from build123d import *

# Parameters (mm, degrees)
F0_W     = 110.9530478716
F0_H     = 111.6942763329
F1_DEPTH = 55.1221389323
F1_TAPER = 3
F2_R     = 10.16
F3_T     = -2.54
F4_R     = 11.5246315094
F4_R_2   = 8.0655463765
F5_DEPTH = 25.4
F6_DEPTH = 25.4


with BuildPart() as f1:
    # F0 (on Top) → F1 (new body)
    with BuildSketch(Plane.XY):
        Rectangle(F0_W, F0_H)
    extrude(amount=F1_DEPTH, taper=F1_TAPER)

    # F2
    f2_edges = [f1.edges().sort_by_distance(p)[0] for p in [
        (54.032109, -54.402724, 27.561069),
        (52.587695, 0, 55.122139),
        (0, -52.958309, 55.122139),
        (54.032109, 54.402724, 27.561069),
        (0, 52.958309, 55.122139),
        (-54.032109, 54.402724, 27.561069),
        (-52.587695, 0, 55.122139),
        (-54.032109, -54.402724, 27.561069),
    ]]
    fillet(f2_edges, radius=F2_R)

    # F3
    f3_openings = [f1.faces().sort_by_distance(p)[0] for p in [
        (0, 0, 0),
    ]]
    offset(amount=F3_T, openings=f3_openings)

    # F4 (on face) → F5 (join)
    with BuildSketch(Plane(origin=(0, 0, 52.5821389323), x_dir=(1, 0, 0), z_dir=(0, 0, -1))):
        with Locations((24.3312865496, -14.7694125772)):
            Circle(F4_R)
        with Locations((24.3312865496, -14.7694125772)):
            Circle(F4_R_2, mode=Mode.SUBTRACT)
    extrude(amount=F5_DEPTH)

    # F6 (cut): a face of the model
    f6_faces = [f1.faces().sort_by_distance(p)[0] for p in [
        (24.3312865496, 14.7694125772, 52.5821389323),
    ]]
    extrude(f6_faces, amount=-F6_DEPTH, mode=Mode.SUBTRACT)


solid = f1.part
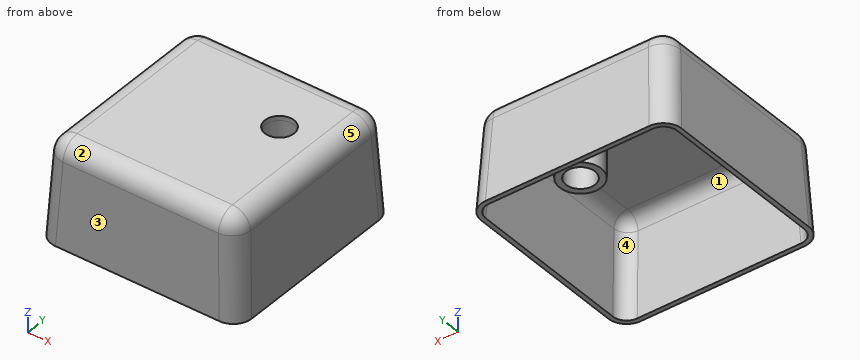
Can you work these out from the model? Positions are in its coordinate system, mm. Face numbers are marked on the shaded views. A direction names the side the tool comes from. Give positions to 0.01 mm unless a question says otherwise; leave off trailing zeros. Order: outer loops, then holes, each group sorted by start corner. A loop starts at its lowest first (then second) coordinate and runs counter-clockwise, first axis right, second up. Notation, with made-up numbers: M -19.5,84.5 L 13.5,84.5 A20 ccw 13.5,105.5 Z; hole C 88.5,45.5 d2. An arc over 180 degrees is marked long. One line per question, with ' | ' between items.
Item 1: For the marked faces 1 and 2, which set-ups out of +Z, -Z, +X, -X, +Y, -Y let a thin tool reach every point of the face, with its end or its side?
Answer block:
face 1: -Z | face 2: +Z, +X, -X, -Y
Item 2: Suppose I cut it at C-C, the plane y = 21. Write out the boundary of the cut face in (x, z).
Answer block:
outline: M -55.48,0 L -52.93,0 L -50.56,45.36 A7.62 cw -42.95,52.58 L 14.64,52.58 L 14.64,27.18 L 19.21,27.18 L 19.21,55.12 L -42.95,55.12 A10.16 ccw -53.09,45.49 Z; M 29.45,27.18 L 34.03,27.18 L 34.03,52.58 L 42.95,52.58 A7.62 cw 50.56,45.36 L 52.93,0 L 55.48,0 L 53.09,45.49 A10.16 ccw 42.95,55.12 L 29.45,55.12 Z
Item 3: Suppose I cut it at B-B, the plane x = -2.5. Write out the boundary of the cut face in (y, z), then the cut area to 3 significant figures.
Answer block:
outline: M -55.85,0 L -53.3,0 L -50.93,45.36 A7.62 cw -43.32,52.58 L 43.32,52.58 A7.62 cw 50.93,45.36 L 53.3,0 L 55.85,0 L 53.46,45.49 A10.16 ccw 43.32,55.12 L -43.32,55.12 A10.16 ccw -53.46,45.49 Z | area: 520 mm2
Item 4: We'd pull the mould along Y, two halves only. Please class the marked faces 3, 4 and 5: released by +Y, released by -Y, zero draft, split by the parting line, or undercut.
Answer block:
face 3: released by -Y | face 4: undercut | face 5: zero draft
Item 5: Suppose I cut it at D-D, the plane y = 40.5. Write out the boundary of the cut face in (x, z), then the cut area to 3 significant figures.
Answer block:
outline: M -55.48,0 L -52.93,0 L -50.56,45.36 A7.62 cw -42.95,52.58 L 42.95,52.58 A7.62 cw 50.56,45.36 L 52.93,0 L 55.48,0 L 53.09,45.49 A10.16 ccw 42.95,55.12 L -42.95,55.12 A10.16 ccw -53.09,45.49 Z | area: 518 mm2
Item 6: Suppose I cut it at A-A, the plane z = 49.5. Write out the boundary of the cut face in (x, y).
Answer block:
outline: M -52.04,-43.32 A9.09 ccw -42.95,-52.41 L 42.95,-52.41 A9.09 ccw 52.04,-43.32 L 52.04,43.32 A9.09 ccw 42.95,52.41 L -42.95,52.41 A9.09 ccw -52.04,43.32 Z; C 24.33,14.77 d23.05; hole M -49.07,-43.32 A6.12 ccw -42.95,-49.44 L 42.95,-49.44 A6.12 ccw 49.07,-43.32 L 49.07,43.32 A6.12 ccw 42.95,49.44 L -42.95,49.44 A6.12 ccw -49.07,43.32 Z; hole C 24.33,14.77 d16.13
Item 7: Please list where these lines run through material, in increasing order: L1, parallel to Y at x = -19, z = 7; L2, parallel to Y at x = 24, z = 41.5; L3, parallel to Z at x = 1, y = 8.
Answer block:
L1: y = -55.48 to -52.94, 52.94 to 55.48 | L2: y = -53.67 to -51.13, 3.25 to 6.71, 22.83 to 26.29, 51.13 to 53.67 | L3: z = 52.58 to 55.12
Item 8: I'm going to push flat-ended pins straight in: pin 1 Ø12 at (x, y) = (-14.5, -16) entering from -Z; pin 2 Ø5 at (x, z) = (-4.5, 18) entering from +Y; pin 3 Ø18.5 at (x, y) = (27, 20.5) entering from -Z. Where does each tip first touch, or does it pass through?
Answer block:
pin 1: stops at z = 52.58 | pin 2: stops at y = 55.03 | pin 3: stops at z = 27.18
